Here's the drawing with two shaded views (mm, measured from the low corner). I have some questions. A direction names the side the tool comes from. Round coordinates to 2 decimals unless told otherwise and drop trailing zeros. Loops run counter-clockwise (first coordinate to the right, second up) from the corner with the lowest first, then second, coordinate; pieces in that order, holes last. Notation, with made-up numbers: M 18,43 L 71,43 A18 ccw 71,73 Z; hole C 47.25,87 d3. An arc over 180 degrees is marked long. Answer as CSV lines item,"result".
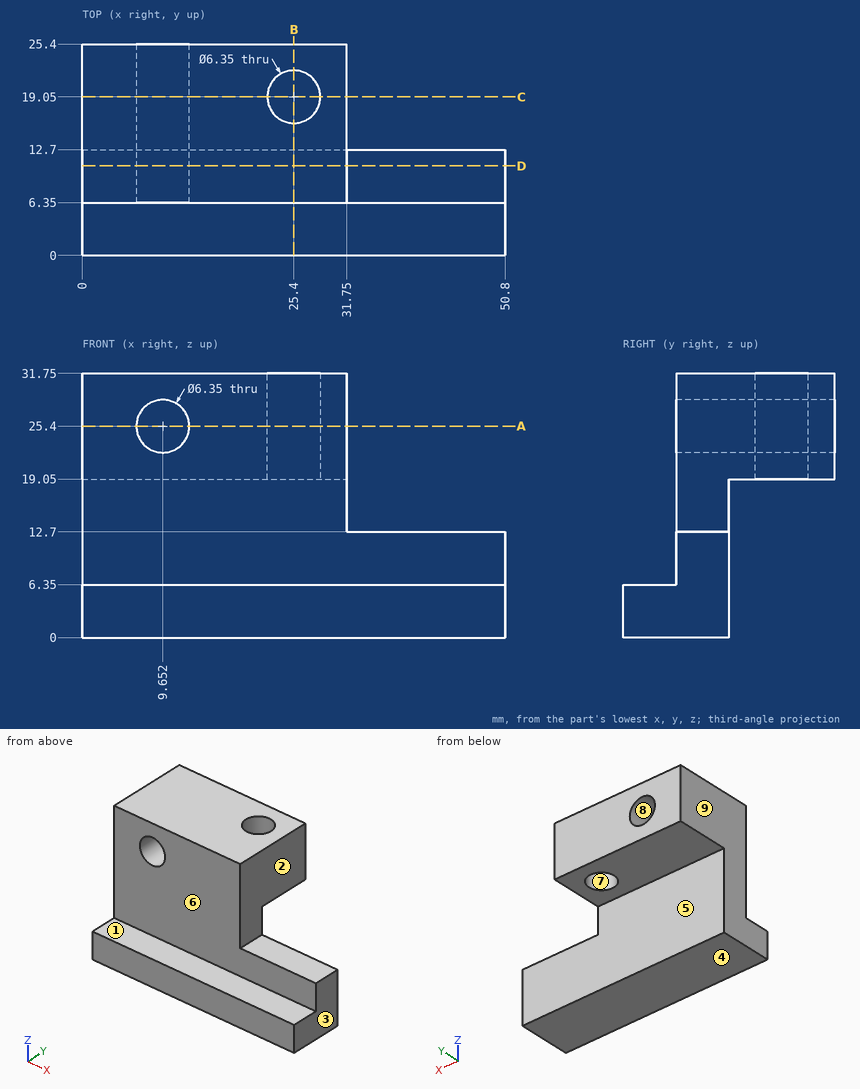
1. I want a section at B-B, the plane x = 25.4. Please give me the cut outline in (y, z) (3 decimals).
Evaluation:
outline,"M 0,0 L 12.7,0 L 12.7,19.05 L 15.875,19.05 L 15.875,31.75 L 6.35,31.75 L 6.35,6.35 L 0,6.35 Z; M 22.225,19.05 L 25.4,19.05 L 25.4,31.75 L 22.225,31.75 Z"
2. Which directions (+Z, -Z, +X, -X, +Y, -Y) give clear straight access to the entire face, cutting with the end or side of a thin tool? Please do the marked faces 1, 2, 3, 4 and 5.
Evaluation:
face 1,"+Z, +X, -X, -Y"
face 2,"+Z, +X, +Y, -Y"
face 3,"+Z, -Z, +X, +Y, -Y"
face 4,"-Z, +X, -X, +Y, -Y"
face 5,"-Z, +X, -X, +Y"
3. I want a section at C-C, the plane y = 19.05. Please give me the cut outline in (x, z) (3 decimals), and give its area (3 significant figures).
Evaluation:
outline,"M 0,19.05 L 22.225,19.05 L 22.225,31.75 L 0,31.75 Z; M 28.575,19.05 L 31.75,19.05 L 31.75,31.75 L 28.575,31.75 Z; hole C 9.652,25.4 d6.35"
area,"291 mm²"
4. I want a section at D-D, the plane y = 10.75. Please give me the cut outline in (x, z) (3 decimals), and give its area (3 significant figures).
Evaluation:
outline,"M 0,0 L 50.8,0 L 50.8,12.7 L 31.75,12.7 L 31.75,31.75 L 0,31.75 Z; hole C 9.652,25.4 d6.35"
area,"1,220 mm²"
5. If I drill on line 1 (X direction, y = 17, z = 25); line 2 (Y direction, x = 25.4, z = 28.75) (3 decimals); line 3 (Z direction, x = 20, y = 3.5), over which ranges is the centre line in solid material (lowest first)? Write a range as [from, to].
Evaluation:
line 1,"x = [0, 6.5], [12.8, 22.98], [27.82, 31.75]"
line 2,"y = [6.35, 15.875], [22.225, 25.4]"
line 3,"z = [0, 6.35]"
6. I want a section at A-A, the plane z = 25.4. Please give me the cut outline in (x, y) (3 decimals), and give its area (3 significant figures).
Evaluation:
outline,"M 0,6.35 L 6.477,6.35 L 6.477,25.4 L 0,25.4 Z; M 12.827,6.35 L 31.75,6.35 L 31.75,25.4 L 12.827,25.4 Z; hole C 25.4,19.05 d6.35"
area,"452 mm²"
7. For P1, Ø12, axis at x = 45, y = 12, coming from the +Z side; P2, Ø6, axis at x = 32, z = 23.5, coming from the +Y side; P3, Ø12.5, axis at x = 18, z = 16.5, coming from the -Y side; P4, Ø9.5, axis at y = 11.5, z = 25.5, coming from the +X side, each with a flat end and sliding along its axis, tell me the tip position at first contact or that it passes through.
Evaluation:
P1,"stops at z = 12.7"
P2,"stops at y = 25.4"
P3,"stops at y = 6.35"
P4,"stops at x = 31.75"
8. We'd pull the mould along X, two halves only. Please class the marked faces 6, 7, 8 and 9: pulls with the +X half, pulls with the -X half, needs draft (parallel to the pull), parting line crosses it, or undercut.
Evaluation:
face 6,"needs draft"
face 7,"undercut"
face 8,"undercut"
face 9,"pulls with the -X half"
